Check sheet for the modelled part. Datum: model origin and axes. Units: mm. Give positions to 0.01 mm unless a question says otherwise; leave off trailing zeros. Loops run counter-clockwise (first coordinate to the right, second up) from the corner with the lowest first, then second, coordinate; pieces in that order, holes last. Notation, with made-up numbers: (4.25, -17.75) -> (26.25, -17.75) arc R11 ccw to (26.25, 2.25) -> close; hole circle Ø6 at (67, 17). An arc over 180 degrees is marked (long way). Write each question's results on one line, items separated by ' | '. Start each with the question number.
Item 1: Gauge pin test, flat ends, axial feed: pin 1 Ø0.8 at (x, z) = (-52, 0.5) entering from -Y; pin 2 Ø0.8 at (y, z) = (-24.5, 1) entering from -X; pin 3 Ø1.1 at (y, z) = (60.5, 0.5) entering from -X. Record the tip position at first contact, or that the pin passes through.
Item 2: Cross-section at B-B on x = 35. Enter the section's corners in (y, z).
Item 3: Cross-section at A-A on y = -42. Enter the section's corners in (x, z).
Item 4: Scan lines: line 1 along Y through (x, z) = (-30, 1.45); line 2 along X through (y, z) = (-9, 0.3); line 3 along X through (y, z) = (-4, 2). Record each from-to range of solid material in increasing order.
Item 5: Cross-section at C-C on z = 2.15. State how many separate pieces and enclosed holes the cut face has, then the cut area to 3 significant figures.
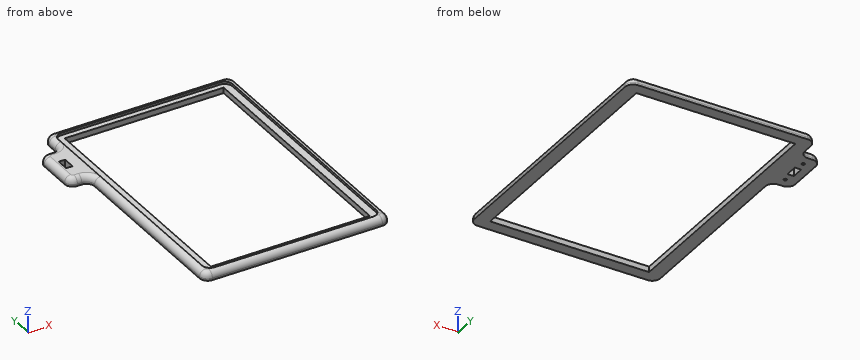
from build123d import *

# Parameters (mm, degrees)
SCHIZZO1_W                   = 3.2
SCHIZZO1_H                   = 6.2
SCHIZZO1_W_2                 = 80
SCHIZZO1_H_2                 = 122
ESTRUSIONE_ESTRUSIONE1_DEPTH = 4
SCHIZZO5_W                   = 80
SCHIZZO5_H                   = 122
TAGLIO_ESTRUSIONE4_DEPTH     = 1.2
SCHIZZO6_R                   = 0.75
TAGLIO_ESTRUSIONE5_DEPTH     = 3
RACCORDO1_R                  = 3


with BuildPart() as part:
    # Schizzo1 → Estrusione-Estrusione1 (new body)
    with BuildSketch(Plane.XY):
        with BuildLine():
            Line((-42.8, -66.9), (42.8, -66.9))
            ThreePointArc((42.8, -66.9), (45.628427125, -65.728427125), (46.8, -62.9))
            Line((46.8, -62.9), (46.8, 62.9))
            ThreePointArc((46.8, 62.9), (45.628427125, 65.728427125), (42.8, 66.9))
            Line((42.8, 66.9), (-42.638118868, 66.9))
            ThreePointArc((-42.638118868, 66.9), (-45.466545993, 65.728427125), (-46.638118868, 62.9))
            Line((-46.638118868, 62.9), (-46.638118868, 57.77646377))
            ThreePointArc((-46.638118868, 57.77646377), (-47.809691743, 54.948036646), (-50.638118868, 53.77646377))
            Line((-50.638118868, 53.77646377), (-53, 53.77646377))
            ThreePointArc((-53, 53.77646377), (-55.828427125, 52.604890895), (-57, 49.77646377))
            Line((-57, 49.77646377), (-57, 32.77646377))
            ThreePointArc((-57, 32.77646377), (-55.828427125, 29.948036646), (-53, 28.77646377))
            Line((-53, 28.77646377), (-50.8, 28.77646377))
            ThreePointArc((-50.8, 28.77646377), (-47.971572875, 27.604890895), (-46.8, 24.77646377))
            Line((-46.8, 24.77646377), (-46.8, -62.9))
            ThreePointArc((-46.8, -62.9), (-45.628427125, -65.728427125), (-42.8, -66.9))
        make_face()
        with Locations((-51.4, 41.27646377)):
            Rectangle(SCHIZZO1_W, SCHIZZO1_H, mode=Mode.SUBTRACT)
        Rectangle(SCHIZZO1_W_2, SCHIZZO1_H_2, mode=Mode.SUBTRACT)
    extrude(amount=ESTRUSIONE_ESTRUSIONE1_DEPTH)

    # Schizzo5 → Taglio-Estrusione4 (cut)
    with BuildSketch(Plane.XY.offset(4)):
        with BuildLine():
            Line((-39.8, 63.9), (39.8, 63.9))
            ThreePointArc((39.8, 63.9), (42.628427125, 62.728427125), (43.8, 59.9))
            Line((43.8, 59.9), (43.8, -59.9))
            ThreePointArc((43.8, -59.9), (42.628427125, -62.728427125), (39.8, -63.9))
            Line((39.8, -63.9), (-39.8, -63.9))
            ThreePointArc((-39.8, -63.9), (-42.628427125, -62.728427125), (-43.8, -59.9))
            Line((-43.8, -59.9), (-43.8, 59.9))
            ThreePointArc((-43.8, 59.9), (-42.628427125, 62.728427125), (-39.8, 63.9))
        make_face()
        Rectangle(SCHIZZO5_W, SCHIZZO5_H, mode=Mode.SUBTRACT)
    extrude(amount=-TAGLIO_ESTRUSIONE4_DEPTH, mode=Mode.SUBTRACT)

    # Schizzo6 → Taglio-Estrusione5 (cut)
    with BuildSketch(Plane(origin=(0, 0, 0), x_dir=(-1, 0, 0), z_dir=(0, 0, -1))):
        with Locations((51.344911825, 48.77646377)):
            Circle(SCHIZZO6_R)
        with Locations((51.344911825, 33.77646377)):
            Circle(SCHIZZO6_R)
    extrude(amount=-TAGLIO_ESTRUSIONE5_DEPTH, mode=Mode.SUBTRACT)

    # Raccordo1
    # the kernel refuses this fillet: 3 mm, written as the material it takes off along each edge
    with BuildSketch(Plane(origin=(-42.8, -66.9, 4), x_dir=(0, 0, -1), z_dir=(1, 0, 0))) as raccordo1_piece_1:
        with BuildLine():
            CenterArc((RACCORDO1_R, RACCORDO1_R), RACCORDO1_R, 180, 90)
            Line((0, RACCORDO1_R), (0, 0))
            Line((0, 0), (RACCORDO1_R, 0))
        make_face()
    extrude(amount=85.6, mode=Mode.SUBTRACT)
    with BuildSketch(Plane(origin=(42.8, -62.9, 4), x_dir=(0, -1, 0), z_dir=(-1, 0, 0))) as raccordo1_piece_2:
        with BuildLine():
            CenterArc((4 - RACCORDO1_R, -RACCORDO1_R), RACCORDO1_R, 0, 90)
            Line((4 - RACCORDO1_R, 0), (4, 0))
            Line((4, 0), (4, -RACCORDO1_R))
        make_face()
    revolve(axis=Axis((42.8, -62.9, 4), (0, 0, 1)), revolution_arc=90, mode=Mode.SUBTRACT)
    with BuildSketch(Plane(origin=(46.8, -62.9, 4), x_dir=(-1, 0, 0), z_dir=(0, 1, 0))) as raccordo1_piece_3:
        with BuildLine():
            CenterArc((RACCORDO1_R, -RACCORDO1_R), RACCORDO1_R, 90, 90)
            Line((0, -RACCORDO1_R), (0, 0))
            Line((0, 0), (RACCORDO1_R, 0))
        make_face()
    extrude(amount=125.8, mode=Mode.SUBTRACT)
    with BuildSketch(Plane(origin=(42.8, 62.9, 4), x_dir=(1, 0, 0), z_dir=(0, -1, 0))) as raccordo1_piece_4:
        with BuildLine():
            CenterArc((4 - RACCORDO1_R, -RACCORDO1_R), RACCORDO1_R, 0, 90)
            Line((4, -RACCORDO1_R), (4, 0))
            Line((4, 0), (4 - RACCORDO1_R, 0))
        make_face()
    revolve(axis=Axis((42.8, 62.9, 4), (0, 0, 1)), revolution_arc=90, mode=Mode.SUBTRACT)
    with BuildSketch(Plane(origin=(42.8, 66.9, 4), x_dir=(0, -1, 0), z_dir=(-1, 0, 0))) as raccordo1_piece_5:
        with BuildLine():
            CenterArc((RACCORDO1_R, -RACCORDO1_R), RACCORDO1_R, 90, 90)
            Line((0, -RACCORDO1_R), (0, 0))
            Line((0, 0), (RACCORDO1_R, 0))
        make_face()
    extrude(amount=85.438118868, mode=Mode.SUBTRACT)
    with BuildSketch(Plane(origin=(-42.638118868, 62.9, 4), x_dir=(0, 1, 0), z_dir=(1, 0, 0))) as raccordo1_piece_6:
        with BuildLine():
            CenterArc((4 - RACCORDO1_R, -RACCORDO1_R), RACCORDO1_R, 0, 90)
            Line((4, -RACCORDO1_R), (4, 0))
            Line((4, 0), (4 - RACCORDO1_R, 0))
        make_face()
    revolve(axis=Axis((-42.638118868, 62.9, 4), (0, 0, 1)), revolution_arc=90, mode=Mode.SUBTRACT)
    with BuildSketch(Plane(origin=(-46.638118868, 62.9, 4), x_dir=(1, 0, 0), z_dir=(0, -1, 0))) as raccordo1_piece_7:
        with BuildLine():
            CenterArc((RACCORDO1_R, -RACCORDO1_R), RACCORDO1_R, 90, 90)
            Line((0, -RACCORDO1_R), (0, 0))
            Line((0, 0), (RACCORDO1_R, 0))
        make_face()
    extrude(amount=5.12353623, mode=Mode.SUBTRACT)
    with BuildSketch(Plane(origin=(-50.638118868, 57.77646377, 4), x_dir=(1, 0, 0), z_dir=(0, 1, 0))) as raccordo1_piece_8:
        with BuildLine():
            CenterArc((4 + RACCORDO1_R, RACCORDO1_R), RACCORDO1_R, 180, 90)
            Line((4, RACCORDO1_R), (4, 0))
            Line((4, 0), (4 + RACCORDO1_R, 0))
        make_face()
    revolve(axis=Axis((-50.638118868, 57.77646377, 4), (0, 0, -1)), revolution_arc=90, mode=Mode.SUBTRACT)
    with BuildSketch(Plane(origin=(-50.638118868, 53.77646377, 4), x_dir=(0, -1, 0), z_dir=(-1, 0, 0))) as raccordo1_piece_9:
        with BuildLine():
            CenterArc((RACCORDO1_R, -RACCORDO1_R), RACCORDO1_R, 90, 90)
            Line((0, -RACCORDO1_R), (0, 0))
            Line((0, 0), (RACCORDO1_R, 0))
        make_face()
    extrude(amount=2.361881132, mode=Mode.SUBTRACT)
    with BuildSketch(Plane(origin=(-53, 49.77646377, 4), x_dir=(0, 1, 0), z_dir=(1, 0, 0))) as raccordo1_piece_10:
        with BuildLine():
            CenterArc((4 - RACCORDO1_R, -RACCORDO1_R), RACCORDO1_R, 0, 90)
            Line((4, -RACCORDO1_R), (4, 0))
            Line((4, 0), (4 - RACCORDO1_R, 0))
        make_face()
    revolve(axis=Axis((-53, 49.77646377, 4), (0, 0, 1)), revolution_arc=90, mode=Mode.SUBTRACT)
    with BuildSketch(Plane(origin=(-57, 49.77646377, 4), x_dir=(1, 0, 0), z_dir=(0, -1, 0))) as raccordo1_piece_11:
        with BuildLine():
            CenterArc((RACCORDO1_R, -RACCORDO1_R), RACCORDO1_R, 90, 90)
            Line((0, -RACCORDO1_R), (0, 0))
            Line((0, 0), (RACCORDO1_R, 0))
        make_face()
    extrude(amount=17, mode=Mode.SUBTRACT)
    with BuildSketch(Plane(origin=(-53, 32.77646377, 4), x_dir=(-1, 0, 0), z_dir=(0, 1, 0))) as raccordo1_piece_12:
        with BuildLine():
            CenterArc((4 - RACCORDO1_R, -RACCORDO1_R), RACCORDO1_R, 0, 90)
            Line((4, -RACCORDO1_R), (4, 0))
            Line((4, 0), (4 - RACCORDO1_R, 0))
        make_face()
    revolve(axis=Axis((-53, 32.77646377, 4), (0, 0, 1)), revolution_arc=90, mode=Mode.SUBTRACT)
    with BuildSketch(Plane(origin=(-53, 28.77646377, 4), x_dir=(0, 1, 0), z_dir=(1, 0, 0))) as raccordo1_piece_13:
        with BuildLine():
            CenterArc((RACCORDO1_R, -RACCORDO1_R), RACCORDO1_R, 90, 90)
            Line((0, -RACCORDO1_R), (0, 0))
            Line((0, 0), (RACCORDO1_R, 0))
        make_face()
    extrude(amount=2.2, mode=Mode.SUBTRACT)
    with BuildSketch(Plane(origin=(-50.8, 24.77646377, 4), x_dir=(0, 1, 0), z_dir=(-1, 0, 0))) as raccordo1_piece_14:
        with BuildLine():
            CenterArc((4 + RACCORDO1_R, RACCORDO1_R), RACCORDO1_R, 180, 90)
            Line((4, RACCORDO1_R), (4, 0))
            Line((4, 0), (4 + RACCORDO1_R, 0))
        make_face()
    revolve(axis=Axis((-50.8, 24.77646377, 4), (0, 0, -1)), revolution_arc=90, mode=Mode.SUBTRACT)
    with BuildSketch(Plane(origin=(-46.8, 24.77646377, 4), x_dir=(1, 0, 0), z_dir=(0, -1, 0))) as raccordo1_piece_15:
        with BuildLine():
            CenterArc((RACCORDO1_R, -RACCORDO1_R), RACCORDO1_R, 90, 90)
            Line((0, -RACCORDO1_R), (0, 0))
            Line((0, 0), (RACCORDO1_R, 0))
        make_face()
    extrude(amount=87.67646377, mode=Mode.SUBTRACT)
    with BuildSketch(Plane(origin=(-42.8, -62.9, 4), x_dir=(-1, 0, 0), z_dir=(0, 1, 0))) as raccordo1_piece_16:
        with BuildLine():
            CenterArc((4 - RACCORDO1_R, -RACCORDO1_R), RACCORDO1_R, 0, 90)
            Line((4 - RACCORDO1_R, 0), (4, 0))
            Line((4, 0), (4, -RACCORDO1_R))
        make_face()
    revolve(axis=Axis((-42.8, -62.9, 4), (0, 0, 1)), revolution_arc=90, mode=Mode.SUBTRACT)


solid = part.part
Answer sheet:
1) pin 1: stops at y = 28.78 | pin 2: stops at x = -46.8 | pin 3: stops at x = -46.64
2) outline: (-66.9, 0) -> (-61, 0) -> (-61, 2.8) -> (-63.9, 2.8) -> (-63.9, 4) arc R3 ccw to (-66.9, 1) -> close; (61, 0) -> (66.9, 0) -> (66.9, 1) arc R3 ccw to (63.9, 4) -> (63.9, 2.8) -> (61, 2.8) -> close
3) outline: (-46.8, 0) -> (-40, 0) -> (-40, 2.8) -> (-43.8, 2.8) -> (-43.8, 4) arc R3 ccw to (-46.8, 1) -> close; (40, 0) -> (46.8, 0) -> (46.8, 1) arc R3 ccw to (43.8, 4) -> (43.8, 2.8) -> (40, 2.8) -> close
4) line 1: y = -66.87 to -61, 61 to 66.87 | line 2: x = -46.8 to -40, 40 to 46.8 | line 3: x = -46.63 to -40, 40 to 46.63
5) separate pieces: 1 | enclosed holes: 4 | area: 2,870 mm²
